```python
from build123d import *

# Parameters (mm, degrees)
SZKIC1_R                    = 20
DODANIE_WYCI_GNI_CIE1_DEPTH = 5
SZKIC2_R                    = 35
SZKIC2_R_2                  = 30
DODANIE_WYCI_GNI_CIE2_DEPTH = 30
ZAOKR_GLENIE1_R             = 3
SFAZOWANIE1_SIZE            = 1
WYTNIJ_WYCI_GNI_CIE1_REACH  = 377.661
SZKIC3_W                    = 40
SZKIC3_H                    = 30


with BuildPart() as part:
    # Szkic1 → Dodanie-wyciągnięcie1 (new body)
    with BuildSketch(Plane.XY):
        with BuildLine():
            Line((184.10343706, -161.91555121), (259.924038765, 268.08444879))
            Line((259.924038765, 268.08444879), (255, 268.952689679))
            Line((255, 268.952689679), (-255, 268.952689679))
            Line((-255, 268.952689679), (-259.924038765, 268.08444879))
            Line((-259.924038765, 268.08444879), (-196.501079187, -91.605028812))
            ThreePointArc((-196.501079187, -91.605028812), (-196.31271073, -92.420942238), (-196.040087999, -93.212696138))
            Line((-196.040087999, -93.212696138), (-145.637863945, -217.962578277))
            ThreePointArc((-145.637863945, -217.962578277), (-144.258069751, -220.214197762), (-142.220393109, -221.89392876))
            Line((-142.220393109, -221.89392876), (-62.568634717, -267.880892909))
            ThreePointArc((-62.568634717, -267.880892909), (-58.568634717, -268.952689679), (-54.568634717, -267.880892909))
            Line((-54.568634717, -267.880892909), (25.977713055, -221.37743734))
            Line((25.977713055, -221.37743734), (24.300392396, -218.442734314))
            Line((24.300392396, -218.442734314), (179.179398295, -161.047310321))
            Line((179.179398295, -161.047310321), (184.10343706, -161.91555121))
        make_face()
        with Locations((18.477713055, -91.047310321)):
            Circle(SZKIC1_R, mode=Mode.SUBTRACT)
    extrude(amount=DODANIE_WYCI_GNI_CIE1_DEPTH)

    # Szkic2 → Dodanie-wyciągnięcie2 (add)
    with BuildSketch(Plane(origin=(0, 0, 0), x_dir=(-1, 0, 0), z_dir=(0, 0, -1))):
        with Locations(Location((-18.477713055, -91.047310321, 0), (0, 0, 180))):
            Circle(SZKIC2_R)
        with Locations((-18.477713055, -91.047310321)):
            Circle(SZKIC2_R_2, mode=Mode.SUBTRACT)
    extrude(amount=DODANIE_WYCI_GNI_CIE2_DEPTH)

    # Zaokrąglenie1
    zaokr_glenie1_edges = [part.edges().sort_by_distance(p)[0] for p in [
        (-16.522286945, -91.047310321, 0),
        (48.477713055, -91.047310321, 0),
    ]]
    fillet(zaokr_glenie1_edges, radius=ZAOKR_GLENIE1_R)

    # Sfazowanie1
    sfazowanie1_edges = [part.edges().sort_by_distance(p)[0] for p in [
        (48.477713055, -91.047310321, -30),
    ]]
    chamfer(sfazowanie1_edges, length=SFAZOWANIE1_SIZE)

    # Wytnij-wyciągnięcie1: up to this face of the body (flat: up to its plane)
    wytnij_wyci_gni_cie1_end = Plane(part.part.faces().sort_by_distance((-2.974035495, 45.126885672, 0))[0])
    # Szkic3 → Wytnij-wyciągnięcie1 (cut, up to the picked face)
    with BuildSketch(Plane(origin=(0, 0, -30), x_dir=(-1, 0, 0), z_dir=(0, 0, -1)), mode=Mode.PRIVATE) as wytnij_wyci_gni_cie1_sk1:
        with Locations((-18.477713055, -60.047310321)):
            Rectangle(SZKIC3_W, SZKIC3_H)
    wytnij_wyci_gni_cie1_tool1 = split(extrude(wytnij_wyci_gni_cie1_sk1.sketch, amount=-WYTNIJ_WYCI_GNI_CIE1_REACH, mode=Mode.PRIVATE), bisect_by=wytnij_wyci_gni_cie1_end, keep=Keep.BOTH, mode=Mode.PRIVATE)
    add(wytnij_wyci_gni_cie1_tool1.solids().sort_by(Axis((18.477713, -60.04731, -30), (0, 0, 1)))[0], mode=Mode.SUBTRACT)


solid = part.part
```
The listing builds one solid part. Answer for the finished solid, in the listing's coordinates (mm). A direction names the side the tool comes from. Round coordinates to 2 decimals unless told otherwise and drop trailing zeros. Order: outer loops, then holes, each group sorted by start corner. A loop starts at its lowest first (then second) coordinate and runs counter-clockwise, first axis right, second up. Notation, with made-up numbers: (-31.75, 42.5) -> (-3.75, 42.5) arc R30 cw to (-3.75, 68.5) -> close; hole circle Ø10 at (-1, -28). An arc over 180 degrees is marked (long way). Answer as CSV lines item,"result". Start each with the question number.
(1) The part is cut by section A-A (z = -20). Determine the outline of the cut face in (x, y), then the cut area to 3 significant figures.
(2) For a pull along Y with two mould halves and no side action, classify faces 1 (the face through (-171.192, -154.714, 2.465)), 2 (the face through (-4, 64, 5)), 3 (the face through (15.87, -71.22, 2.46)) as +Y half, -Y half, draft (parallel to the pull), parting line (faces both ways), or undercut.
(3) Flat-ended cylindrical pins translate along their axes: pin 1 Ø10 at (y, z) = (33, -1.5) entering from +X; pin 2 Ø4.5 at (y, z) = (-69, -12.5) entering from +X; pin 3 Ø4 at (x, y) = (-127, -54.5) entering from -Z. Find the tip coordinate at first contact, or state that the pin passes through.
(4) A tool of negligible diameter and unlimited length cuts with its end or side. For faces 4 (the face through (18, -123, -30)), 5 (the face through (19.49, -121.03, -15.82)), 6 (the face through (38.478, -64, -15)), from which of +Z, -Z, +X, -X, +Y, -Y can it reach the whole face along a straight path? Write none if from no direction.
(5) Find the intervals of material crossed by probe 1 along X at (y, z) = (-89.5, -14); probe 2 along Z at (x, y) = (54, 117); probe 3 along X at (y, z) = (-103, -8.5), in increasing order. Write a range as from..to.
(6) The part is cut by section B-B (x = 195). Determine the outline of the cut face in (y, z), then the cut area to 3 significant figures.
Evaluation:
1,outline,"(-1.52, -68.69) -> (-1.52, -62.32) arc R35 ccw (long way) to (38.48, -62.32) -> (38.48, -68.69) arc R30 cw (long way) to start"
1,area,"805 mm²"
2,face 1,"-Y half"
2,face 2,"draft"
2,face 3,"undercut"
3,pin 1,"x = 219.31"
3,pin 2,"x = 47.34"
3,pin 3,"z = 0"
4,face 4,"-Z, +X, -X, +Y, -Y"
4,face 5,"-Z"
4,face 6,"-Z, +Y"
5,probe 1,"-16.49..-11.48, 48.44..53.44"
5,probe 2,"0..5"
5,probe 3,"-14.42..-9.04, 45.99..51.37"
6,outline,"(-100.12, 0) -> (268.95, 0) -> (268.95, 5) -> (-100.12, 5) -> close"
6,area,"1,850 mm²"
